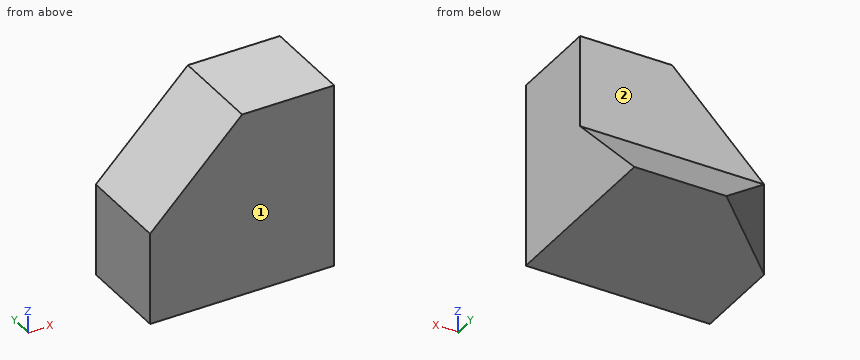
from build123d import *

# Parameters (mm, degrees)
SKETCH1_W           = 40
SKETCH1_H           = 40
BOSS_EXTRUDE1_DEPTH = 40
CUT_EXTRUDE1_DEPTH  = 40
CUT_EXTRUDE2_DEPTH  = 40
CUT_EXTRUDE3_DEPTH  = 40


with BuildPart() as part:
    # Sketch1 → Boss-Extrude1 (new body)
    with BuildSketch(Plane.XY):
        with Locations((20, 20)):
            Rectangle(SKETCH1_W, SKETCH1_H)
    extrude(amount=BOSS_EXTRUDE1_DEPTH)

    # Sketch2 → Cut-Extrude1 (cut)
    with BuildSketch(Plane.XY.offset(40)):
        Polygon((0, 20), (0, 40), (20, 40), align=None)
    extrude(amount=-CUT_EXTRUDE1_DEPTH, mode=Mode.SUBTRACT)

    # Sketch3 → Cut-Extrude2 (cut)
    with BuildSketch(Plane.ZY):
        Polygon((40, 20), (20, 20), (0, 40), (40, 40), align=None)
    extrude(amount=-CUT_EXTRUDE2_DEPTH, mode=Mode.SUBTRACT)

    # Sketch4 → Cut-Extrude3 (cut)
    with BuildSketch(Plane(origin=(0, 20, 0), x_dir=(1, 0, 0), z_dir=(0, 1, 0))):
        Polygon((0, -20), (20, -40), (0, -40), align=None)
    extrude(amount=-CUT_EXTRUDE3_DEPTH, mode=Mode.SUBTRACT)


solid = part.part
Read the model definition and answer for the solid it produces. Units are mm, in the model's axes. Face numbers are marked on the shaded views. A direction names the side the tool comes from. Give positions to 0.01 mm unless a question says otherwise; leave off trailing zeros. Loops run counter-clockwise (first coordinate to the right, second up) from the corner with the lowest first, then second, coordinate; pieces in that order, holes last. Notation, with made-up numbers: (13.25, 37.5) - (55.25, 37.5) arc R17 ccw to (55.25, 42.5) - close; hole circle Ø8 at (71, 89). An arc over 180 degrees is marked (long way). Answer as CSV lines item,"result". Start each with the question number.
1) Which of the six approach directions +Z, -Z, +X, -X, +Y, -Y give full straight-line access (tool end or side, diameter ignored) to the marked faces 1 and 2?
2) Straight lines are drawn through the part: L1, parallel to Y at x = 19, z = 24.5; L2, parallel to Z at x = 11.5, y = 4; L3, parallel to Z at x = 27, y = 28. For each, find the intervals that lie inside material, in ascending order. Write a range as from..to.
3) Find section B-B (x = 34). Write down the section's boundary in (y, z).
4) Find section A-A (z = 17.5). Write down the section's boundary in (x, y).
5) Find section D-D (z = 29). Write down the section's boundary in (x, y).
6) Find section C-C (y = 29.5). Write down the section's boundary in (x, z), then the cut area to 3 significant figures.
7) Each of these flat-tipped pins is pushed along its axis until it touches: pin 1 Ø12 at (x, z) = (30, 18) entering from +Y; pin 2 Ø8 at (x, z) = (33.5, 8) entering from +Y; pin 3 Ø4 at (x, y) = (5.5, 9) entering from +Z. Where does it stop, or does it pass through?
Findings below:
1,face 1,"+Z, -Z, +X, -X, -Y"
1,face 2,"+Z, +X, -X, +Y"
2,L1,"0..20"
2,L2,"0..31.5"
2,L3,"0..12"
3,outline,"(0, 0) - (40, 0) - (20, 20) - (20, 40) - (0, 40) - close"
4,outline,"(0, 0) - (40, 0) - (40, 22.5) - (2.5, 22.5) - (0, 20) - close"
5,outline,"(9, 0) - (40, 0) - (40, 20) - (9, 20) - close"
6,outline,"(9.5, 0) - (40, 0) - (40, 10.5) - (9.5, 10.5) - close"
6,area,"320 mm^2"
7,pin 1,"y = 28"
7,pin 2,"y = 36"
7,pin 3,"z = 27.5"
